```python
from build123d import *

# Parameters (mm, degrees)
SKETCH14_R           = 30.5
BOSS_EXTRUDE11_DEPTH = 39.4589
SKETCH15_R           = 22
CUT_EXTRUDE2_DEPTH   = 59.459428574
SKETCH13_R           = 26.9875
CUT_EXTRUDE3_DEPTH   = 26.9875


with BuildPart() as part:
    # Sketch14 → Boss-Extrude11 (new body)
    with BuildSketch(Plane(origin=(0, 0, 0), x_dir=(0, 0, -1), z_dir=(1, 0, 0))):
        Circle(SKETCH14_R)
    extrude(amount=BOSS_EXTRUDE11_DEPTH)

    # Sketch15 → Cut-Extrude2 (cut, through all)
    with BuildSketch(Plane.ZY):
        Circle(SKETCH15_R)
    extrude(amount=-CUT_EXTRUDE2_DEPTH, mode=Mode.SUBTRACT)

    # Sketch13 → Cut-Extrude3 (cut)
    with BuildSketch(Plane.ZY):
        Circle(SKETCH13_R)
    extrude(amount=-CUT_EXTRUDE3_DEPTH, mode=Mode.SUBTRACT)


solid = part.part
```
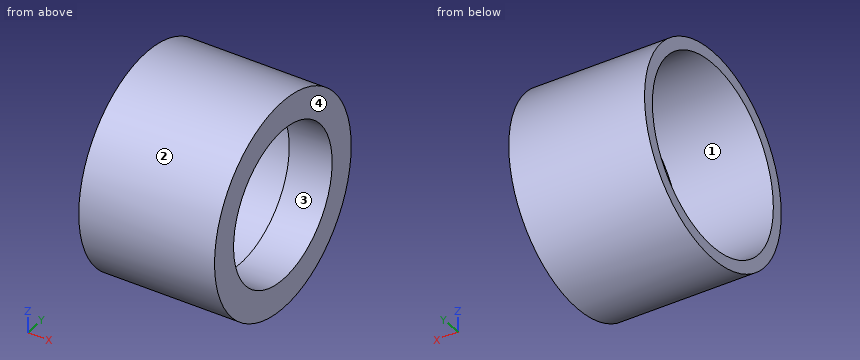
Geometry: final body of the model. Coordinates: model frame, mm. Face numbers are marked on the shaded views. Coordinates: 2 decimals unless noted, no trailing zeros. Write each loop counter-clockwise with the first axis right and the second up, starting at its lowest first coordinate (ties: lowest second). Pieces come first, ordered by that corner, then holes. Notation, with made-up numbers: M 35.25,14.25 L 74.25,14.25 A24 cw 74.25,50.25 Z; hole C 86.25,35.25 d4. An arc over 180 degrees is marked long. Use CSV: the item, a comma, the result in double quotes. Start each with the question number.
1. Cut plane A-A on y = 0. Return the cut outline in (x, z), plus the area to 3 significant figures.
2. Mould query, pull axis Z, two halves, no side actions, for the marked faces 1, 2, 3 and 4. Classes: pulls with the +Z half, pulls with the -Z half, needs draft (parallel to the pull), parting line crosses it, or undercut.
3. Cut plane C-C on x = 32.5. Return the cut outline in (y, z).
4. Cut plane D-D on z = 24.5. Return the cut outline in (x, y).
5. Ray query, probe 1 along Y at (x, z) = (33, 0); probe 2 along Y at (x, z) = (21.5, 0); probe 3 along X at (y, z) = (25, 6). Return the intervals inside material, ascending.
6. First-contact query: P1, Ø5, axis at x = 6.5, y = -17.5, coming from the -Z side; P2, Ø2, axis at x = 26, y = -21, coming from the -Z side; P3, Ø5, axis at x = 16, y = 19, coming from the +Z side. Flat tips, straight axial feed; report the tip coordinate or a pass-through.
Entries:
1,outline,"M 0,-30.5 L 39.46,-30.5 L 39.46,-22 L 26.99,-22 L 26.99,-26.99 L 0,-26.99 Z; M 0,26.99 L 26.99,26.99 L 26.99,22 L 39.46,22 L 39.46,30.5 L 0,30.5 Z"
1,area,"402 mm²"
2,face 1,"undercut"
2,face 2,"parting line crosses it"
2,face 3,"undercut"
2,face 4,"needs draft"
3,outline,"C 0,0 d61; hole C 0,0 d44"
4,outline,"M 0,-18.17 L 39.46,-18.17 L 39.46,18.17 L 0,18.17 L 0,11.32 L 26.99,11.32 L 26.99,-11.32 L 0,-11.32 Z"
5,probe 1,"-30.5 to -22, 22 to 30.5"
5,probe 2,"-30.5 to -26.99, 26.99 to 30.5"
5,probe 3,"26.99 to 39.46"
6,P1,"z = -26.56"
6,P2,"z = -23.03"
6,P3,"z = 25.65"
